Read the model definition and answer for the solid it produces. Units are mm, in the model's axes. Face numbers are marked on the shaded views. A direction names the side the tool comes from. Coordinates: 2 decimals unless noted, no trailing zeros. Order: outer loops, then holes, each group sorted by start corner. A loop starts at its lowest first (then second) coordinate and runs counter-clockwise, first axis right, second up.
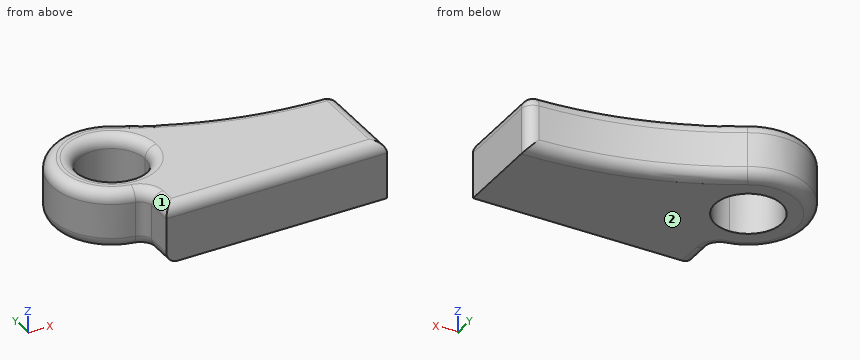
```python
from build123d import *

# Parameters (mm, degrees)
F1_DEPTH = 25
F3_R     = 5


# Not quite as in the source:
# - the program builds the solid bodies; features that only make, move or delete a surface that nothing else refers to are left out


with BuildPart() as f1:
    # F0 (on Top) → F1 (new body)
    with BuildSketch(Plane.XY):
        with BuildLine():
            Line((-22.0192338504, 20.8813082427), (47.958523035, 20.8813082427))
            ThreePointArc((47.958523035, 20.8813082427), (5.048852146, 26.5810643591), (-34.884897805, 43.2850366545))
            ThreePointArc((-34.884897805, 43.2850366545), (-25.4644430478, 33.7988578917), (-22.0192338504, 20.8813082427))
        make_face()
        with BuildLine():
            ThreePointArc((-34.884897805, 43.2850366545), (-72.9983264837, 27.652937785), (-47.958523035, -5.057980942))
            Line((-47.958523035, -5.057980942), (-47.958523035, 6.3973983269))
            ThreePointArc((-47.958523035, 6.3973983269), (-58.2001939546, 31.1229791622), (-33.4746131192, 20.8813082427))
            Line((-33.4746131192, 20.8813082427), (-22.0192338504, 20.8813082427))
            ThreePointArc((-22.0192338504, 20.8813082427), (-25.4644430478, 33.7988578917), (-34.884897805, 43.2850366545))
        make_face()
        with BuildLine():
            Line((-47.958523035, 6.3973983269), (-47.958523035, -5.057980942))
            ThreePointArc((-47.958523035, -5.057980942), (-29.6166757534, 2.539460961), (-22.0192338504, 20.8813082427))
            Line((-22.0192338504, 20.8813082427), (-33.4746131192, 20.8813082427))
            ThreePointArc((-33.4746131192, 20.8813082427), (-37.7168521155, 10.6396373231), (-47.958523035, 6.3973983269))
        make_face()
        with BuildLine():
            Line((-47.958523035, -5.057980942), (-47.958523035, -20.8813082427))
            Line((-47.958523035, -20.8813082427), (47.958523035, -20.8813082427))
            Line((47.958523035, -20.8813082427), (47.958523035, 20.8813082427))
            Line((47.958523035, 20.8813082427), (-22.0192338504, 20.8813082427))
            ThreePointArc((-22.0192338504, 20.8813082427), (-29.6166757534, 2.539460961), (-47.958523035, -5.057980942))
        make_face()
    extrude(amount=-F1_DEPTH)

    # F3
    f3_edges = [f1.edges().sort_by_distance(p)[0] for p in [
        (5.048852, 26.581064, 0),
        (-72.998326, 27.652938, 0),
        (-47.958523, -12.969645, 0),
        (0, -20.881308, 0),
        (47.958523, 0, 0),
        (-62.442433, 20.881308, 0),
        (47.958523, 20.881308, -12.5),
        (-34.884898, 43.285037, -12.5),
        (5.048852, 26.581064, -25),
        (-47.958523, -5.057981, -12.5),
        (-72.998326, 27.652938, -25),
        (-47.958523, -12.969645, -25),
    ]]
    fillet(f3_edges, radius=F3_R)


solid = f1.part
```
1) Flat-ended cylindrical pins translate along their axes: pin 1 Ø12.5 at (y, z) = (-16.5, -10) entering from -X; pin 2 Ø3 at (x, z) = (-31.5, -6.5) entering from +Y; pin 3 Ø5 at (x, z) = (-44.5, -8) entering from +Y. Find the tip coordinate at first contact, or state that the pin passes through.
A:
pin 1: stops at x = -47.96
pin 2: stops at y = 42.2
pin 3: stops at y = 46.8
2) Which of the six approach directions +Z, -Z, +X, -X, +Y, -Y give full straight-line access (tool end or side, diameter ignored) to the marked faces 1 and 2?
A:
face 1: +Z, -X, -Y
face 2: -Z, +X, -X, +Y, -Y
3) Straight lines are drawn through the part: line 1 (X direction, y = 12, z = -17); line 2 (X direction, y = 20.5, z = -9.5) (3 decimals); line 3 (Y direction, x = -40, z = -15.25). For each, find the intervals that lie inside material, in ascending order.
A:
line 1: x = -72.33 to -59.4, -36.52 to 47.96
line 2: x = -73.895 to -62.437, -33.48 to 45.043
line 3: y = -20.88 to 8.78, 32.98 to 45.57
4) A cutting plane is placed at A-A, the plane z = -15.25. Determine the outline of the cut face in (x, y), and give its area (3 significant figures).
A:
outline: (-52.15, -4.72) arc R5 cw to (-47.96, -9.65) - (-47.96, -20.88) - (47.96, -20.88) - (47.96, 15.96) arc R5 ccw to (43.11, 20.95) arc R164.37 cw to (-34.88, 43.29) arc R25.94 ccw (long way) to start; hole circle Ø28.97 at (-47.96, 20.88)
area: 5,330 mm2
